Here's the drawing with two shaded views (mm, measured from the low corner). I have some questions. A direction names the side the tool comes from. Coordinates: 2 decimals unless noted, no trailing zeros. Write each loop counter-clockwise with the first axis right and the second up, starting at its lowest first coordinate (ties: lowest second). Pieces come first, ordered by that corner, then holes.
Item 1: If we section it at D-D (x = 52): Please give me the cut outline in (y, z).
Item 2: I'm going to push flat-ended pins straight in: pin 1 Ø2.5 at (x, z) = (53.5, 4) entering from +Y; pin 2 Ø6 at (x, z) = (57, 14.5) entering from +Y; pin 3 Ø5 at (x, z) = (60, 53.5) entering from -Y. Where does each tip first touch, or does it pass through?
Item 3: We'd pull the mould along X, two halves only. Please class the marked faces 1, 2 and 3: +X half, -X half, draft (parallel to the pull), parting line (faces both ways), or undercut.
Item 4: If we section it at A-A (y = 6.75): Please give me the cut outline in (x, z), then the cut area to 3 significant figures.
Item 5: If we section it at B-B (z = 44.5): Please give me the cut outline in (x, y), then the cut area to 3 significant figures.
Item 6: If I drill on line 1 (Z direction, x = 41.5, y = 5.5); line 2 (Z direction, x = 88.5, y = 15.25); line 3 (X direction, y = 13.5, z = 47.5), over which ranges is the centre line in solid material (lowest first)?
Item 7: If we section it at C-C (y = 19.75): Please give me the cut outline in (x, z), then the cut area to 3 significant figures.
Item 8: For the marked faces 4 and 5, which set-ups out of +Z, -Z, +X, -X, +Y, -Y let a thin tool reach every point of the face, with its end or its side?
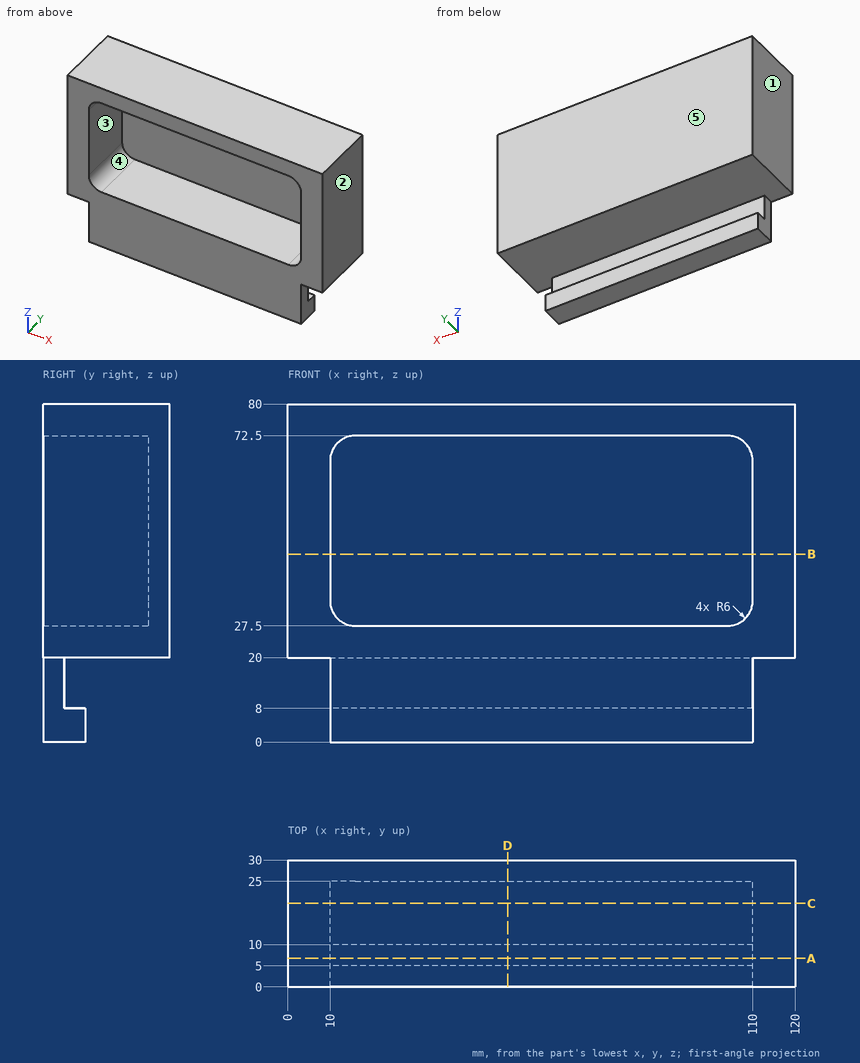
Answer list:
1. outline: (0, 0) - (10, 0) - (10, 8) - (5, 8) - (5, 20) - (30, 20) - (30, 80) - (0, 80) - (0, 72.5) - (25, 72.5) - (25, 27.5) - (0, 27.5) - close
2. pin 1: stops at y = 10
2. pin 2: stops at y = 5
2. pin 3: stops at y = 25
3. face 1: -X half
3. face 2: +X half
3. face 3: undercut
4. outline: (0, 20) - (120, 20) - (120, 80) - (0, 80) - close; (10, 0) - (110, 0) - (110, 8) - (10, 8) - close; hole (10, 33.5) arc R6 ccw to (16, 27.5) - (104, 27.5) arc R6 ccw to (110, 33.5) - (110, 66.5) arc R6 ccw to (104, 72.5) - (16, 72.5) arc R6 ccw to (10, 66.5) - close
4. area: 3,530 mm2
5. outline: (0, 0) - (10, 0) - (10, 25) - (110, 25) - (110, 0) - (120, 0) - (120, 30) - (0, 30) - close
5. area: 1,100 mm2
6. line 1: z = 0 to 8, 20 to 27.5, 72.5 to 80
6. line 2: z = 20 to 27.5, 72.5 to 80
6. line 3: x = 0 to 10, 110 to 120
7. outline: (0, 20) - (120, 20) - (120, 80) - (0, 80) - close; hole (10, 33.5) arc R6 ccw to (16, 27.5) - (104, 27.5) arc R6 ccw to (110, 33.5) - (110, 66.5) arc R6 ccw to (104, 72.5) - (16, 72.5) arc R6 ccw to (10, 66.5) - close
7. area: 2,730 mm2
8. face 4: -Y
8. face 5: +Z, -Z, +X, -X, +Y
